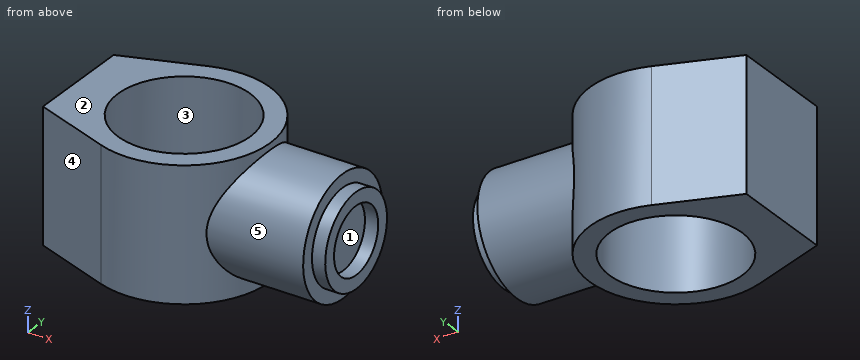
```python
from build123d import *

# Parameters (mm, degrees)
SKETCH_1_R      = 50
EXTRUDE_1_DEPTH = 50
EXTRUDE_2_REACH = 202
SKETCH_2_R      = 45
SKETCH_3_R      = 35
SKETCH_3_R_2    = 25
EXTRUDE_3_DEPTH = 10


with BuildPart() as part:
    # 草图1 → 凸台-拉伸1 (new body, symmetric)
    with BuildSketch(Plane.XY):
        with BuildLine():
            Line((-80, 40), (-80, -40))
            Line((-80, -40), (-22.281665693, -61.061668614))
            ThreePointArc((-22.281665693, -61.061668614), (65, 0), (-22.281665693, 61.061668614))
            Line((-22.281665693, 61.061668614), (-80, 40))
        make_face()
        Circle(SKETCH_1_R, mode=Mode.SUBTRACT)
    extrude(amount=EXTRUDE_1_DEPTH, both=True)

    # 草图2 → 凸台-拉伸2 (add, up to next)
    with BuildSketch(Plane(origin=(120, 0, 0), x_dir=(0, 0, -1), z_dir=(1, 0, 0)), mode=Mode.PRIVATE) as extrude_2_sk1:
        Circle(SKETCH_2_R)
    extrude_2_tool1 = extrude(extrude_2_sk1.sketch, amount=-EXTRUDE_2_REACH, mode=Mode.PRIVATE) - part.part
    add(extrude_2_tool1.solids().sort_by_distance((120, 0, 0))[0])

    # 草图3 → 凸台-拉伸3 (add)
    with BuildSketch(Plane(origin=(120, 0, 0), x_dir=(0, 0, -1), z_dir=(1, 0, 0))):
        Circle(SKETCH_3_R)
        Circle(SKETCH_3_R_2, mode=Mode.SUBTRACT)
    extrude(amount=EXTRUDE_3_DEPTH)


solid = part.part
```
Work out the finished part from the listing and answer in its coordinate system (mm). Face numbers are marked on the shaded views. A direction names the side the tool comes from. Give positions to 0.01 mm unless a question says otherwise; leave off trailing zeros. Loops run counter-clockwise (first coordinate to the right, second up) from the corner with the lowest first, then second, coordinate; pieces in that order, holes last. Notation, with made-up numbers: M 60,71 L 89,71 A26 cw 89,86 Z; hole C -33.75,62 d9. An arc over 180 degrees is marked long. One line per item, written item: value. Start each with the question number.
1. Find section A-A (x = 0). Give the vertices of the cut face in (y, z), and give its area (3 significant figures).
2. Find section C-C (z = 0). Give the vertices of the cut face in (x, y), and give its area (3 significant figures).
3. Find section B-B (y = 0). Give the vertices of the cut face in (x, z), and give its area (3 significant figures).
4. Each of these flat-tipped pins is pushed along its axis until it touches: P1, Ø10, axis at x = 11.5, z = 21, coming from the +Y side; P2, Ø15, axis at y = 6, z = -8, coming from the +X side; P3, Ø5, axis at x = 78, z = -4, coming from the +Y side (3 decimals). Where does it stop, or does it pass through?
5. Find section D-D (x = -30). Give the vertices of the cut face in (y, z), and give its area (3 significant figures).
6. Determine the mould class of the marked faces 1, 2 and 3 for opening direction X: released by +X, released by -X, zero draft, split by the parting line, or undercut.
7. Which of the six approach directions +Z, -Z, +X, -X, +Y, -Y give full straight-line access (tool end or side, diameter ignored) to the marked faces 4 and 5?
8. Find the intervals of material crossed by probe 1 along Y at (x, z) = (0, -28.5); probe 2 along Y at (x, z) = (123, 0); probe 3 along X at (y, z) = (-22, 14), in increasing order.
Reported:
1. outline: M -65,-50 L -50,-50 L -50,50 L -65,50 Z; M 50,-50 L 65,-50 L 65,50 L 50,50 Z
1. area: 3,000 mm²
2. outline: M -80,-40 L -22.28,-61.06 A65 ccw 46.9,-45 L 120,-45 L 120,-35 L 130,-35 L 130,-25 L 120,-25 L 120,25 L 130,25 L 130,35 L 120,35 L 120,45 L 46.9,45 A65 ccw -22.28,61.06 L -80,40 Z; hole C 0,0 d100
2. area: 13,100 mm²
3. outline: M -80,-50 L -50,-50 L -50,50 L -80,50 Z; M 50,-50 L 65,-50 L 65,-45 L 120,-45 L 120,-35 L 130,-35 L 130,-25 L 120,-25 L 120,25 L 130,25 L 130,35 L 120,35 L 120,45 L 65,45 L 65,50 L 50,50 Z
3. area: 9,650 mm²
4. P1: stops at y = 64.67
4. P2: stops at x = 120
4. P3: stops at y = 44.975
5. outline: M -58.25,-50 L -40,-50 L -40,50 L -58.25,50 Z; M 40,-50 L 58.25,-50 L 58.25,50 L 40,50 Z
5. area: 3,650 mm²
6. face 1: released by +X
6. face 2: zero draft
6. face 3: undercut
7. face 4: +Z, -Z, -X, -Y
7. face 5: +X
8. probe 1: y = -65 to -50, 50 to 65
8. probe 2: y = -35 to -25, 25 to 35
8. probe 3: x = -80 to -44.9, 44.9 to 130
